The model under review builds one solid part; all positions refer to its coordinate system, in mm. Face numbers are marked on the shaded views. A direction names the side the tool comes from. Coordinates: 2 decimals unless noted, no trailing zeros. Loops run counter-clockwise (first coordinate to the right, second up) from the corner with the lowest first, then second, coordinate; pieces in that order, holes last. Notation, with made-up numbers: (48.5, 0.5) - (74.5, 0.5) arc R23 cw to (74.5, 31.5) - close; hole circle Ø10 at (82, -4). An arc over 180 degrees is marked (long way). Use a Markdown table: item, result. Add a question column.
1) Add section A-A, the plane z = 13. Give the boundary of the cut face in (x, y).
2) Clearance check with flat-ended pins moving along their axes: pin 1 (4 mm diameter, centred on x = -72.5, z = 28.5, fed in from +Y); pin 2 (10 mm diameter, centred on y = -45.5, z = 17, fed in from +X); pin 3 (6 mm diameter, centred on x = -50.5, y = -45.5, fed in from -Z). State where each tip first meets the part, or that it passes through.
3) The part is to be moulded in two halves that separate along X. For the marked faces 4, 5 and 6, say which applies: pulls with the +X half, pulls with the -X half, needs draft (parallel to the pull), parting line crosses it, or undercut.
4) Add section C-C, the plane x = -36. Give the boundary of the cut face in (y, z), and give its area (3 significant figures).
5) For the marked faces 1, 2 and 3, list the 3-axis set-ups (+Z, -Z, +X, -X, +Y, -Y) from which the entire face can be reached by the end or side of a thin tool; tool diameter is ignored.
6) Add section B-B, the plane y = -39.5. Give the boundary of the cut face in (x, z).
7) To check wall thickness, follow L1, parallel to X at y = -18, z = 38.5; L2, parallel to Y at x = -11, z = 54; L3, parallel to Z at x = -85.5, y = -53. State the ranges of each line that lie inside material, in increasing order. Write a range as [from, to].
8) Add section D-D, the plane x = -21.5. Give the boundary of the cut face in (y, z), and give its area (3 significant figures).
```python
from build123d import *

# Parameters (mm, degrees)
F1_DEPTH = 60
F2_W     = 90
F2_H     = 10
F3_DEPTH = 12
F4_W     = 14
F4_H     = 10
F5_DEPTH = 48
F6_W     = 14
F6_H     = 10
F7_DEPTH = 48


with BuildPart() as f1:
    # F0 (on Front) → F1 (new body)
    with BuildSketch(Plane.XZ):
        Polygon((-90, 0), (0, 0), (0, 10), (-10, 10), (-10, 58), (-24, 58), (-24, 10), (-66, 10), (-66, 58), (-80, 58), (-80, 10), (-90, 10), align=None)
    extrude(amount=F1_DEPTH)

    # F2 (on face) → F3 (join)
    with BuildSketch(Plane(origin=(0, 0, 0), x_dir=(1, 0, 0), z_dir=(0, 0, -1))):
        with Locations((-45, 5)):
            Rectangle(F2_W, F2_H)
    extrude(amount=F3_DEPTH)

    # F4 (on face) → F5 (cut)
    with BuildSketch(Plane.XY.offset(58)):
        with Locations((-17, -5)):
            Rectangle(F4_W, F4_H)
    extrude(amount=-F5_DEPTH, mode=Mode.SUBTRACT)

    # F6 (on face) → F7 (cut)
    with BuildSketch(Plane.XY.offset(58)):
        with Locations((-73, -5)):
            Rectangle(F6_W, F6_H)
    extrude(amount=-F7_DEPTH, mode=Mode.SUBTRACT)


solid = f1.part
```
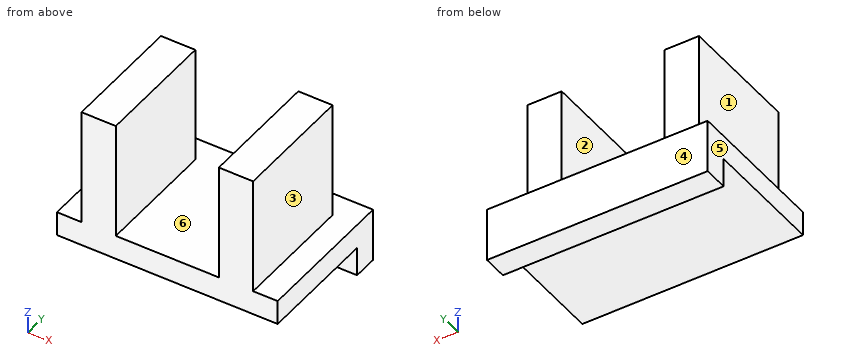
From the geometry:
| question | item | result |
|---|---|---|
| 1 | outline | (-80, -60) - (-66, -60) - (-66, -10) - (-80, -10) - close; (-24, -60) - (-10, -60) - (-10, -10) - (-24, -10) - close |
| 2 | pin 1 | stops at y = -10 |
| 2 | pin 2 | stops at x = -10 |
| 2 | pin 3 | stops at z = 0 |
| 3 | face 4 | needs draft |
| 3 | face 5 | pulls with the -X half |
| 3 | face 6 | undercut |
| 4 | outline | (-60, 0) - (-10, 0) - (-10, -12) - (0, -12) - (0, 10) - (-60, 10) - close |
| 4 | area | 720 mm^2 |
| 5 | face 1 | +Z, -X, +Y, -Y |
| 5 | face 2 | +Z, +Y, -Y |
| 5 | face 3 | +Z, +X, +Y, -Y |
| 6 | outline | (-90, 0) - (0, 0) - (0, 10) - (-10, 10) - (-10, 58) - (-24, 58) - (-24, 10) - (-66, 10) - (-66, 58) - (-80, 58) - (-80, 10) - (-90, 10) - close |
| 7 | L1 | x = [-80, -66], [-24, -10] |
| 7 | L2 | y = [-60, -10] |
| 7 | L3 | z = [0, 10] |
| 8 | outline | (-60, 0) - (-10, 0) - (-10, -12) - (0, -12) - (0, 10) - (-10, 10) - (-10, 58) - (-60, 58) - close |
| 8 | area | 3,120 mm^2 |
